Print and shaded views of the part. All mm, measured from the part's lowest x, y and z. A direction names the side the tool comes from. Round coordinates to 2 decimals unless told otherwise and drop trailing zeros. Order: outer loops, then holes, each group sorted by start corner. A loop starts at its lowest first (then second) coordinate and runs counter-clockwise, first axis right, second up. Notation, with made-up numbers: (-22, 42.25) - (35, 42.25) arc R21 cw to (35, 67.25) - close; hole circle Ø1 at (-36.5, 77). An arc over 180 degrees is marked (long way). Write item = value, one per line.
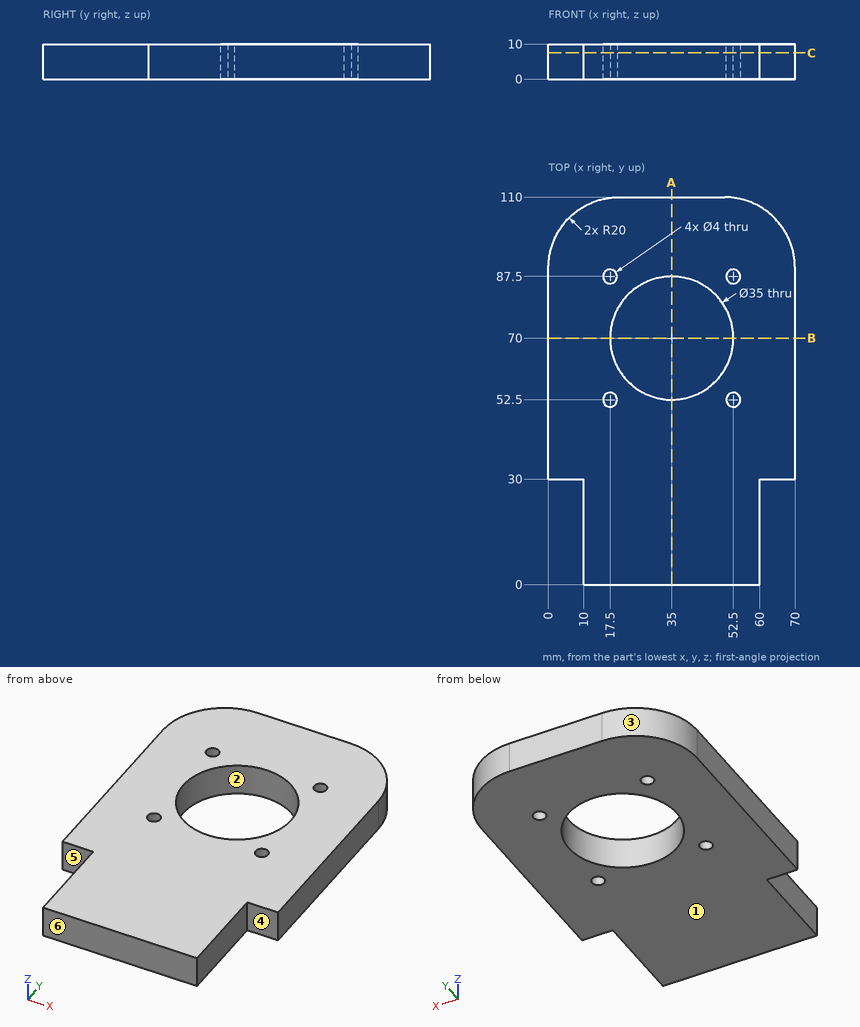
(1) Band-saw the part on B-B on y = 70. List the corners of the cut face in (x, z), plus the area to 3 significant figures.
Solved:
outline = (0, 0) - (17.5, 0) - (17.5, 10) - (0, 10) - close; (52.5, 0) - (70, 0) - (70, 10) - (52.5, 10) - close
area = 350 mm²
(2) Band-saw the part on C-C on z = 7.5. List the corners of the cut face in (x, y).
Solved:
outline = (0, 30) - (10, 30) - (10, 0) - (60, 0) - (60, 30) - (70, 30) - (70, 90) arc R20 ccw to (50, 110) - (20, 110) arc R20 ccw to (0, 90) - close; hole circle Ø4 at (17.5, 52.5); hole circle Ø4 at (17.5, 87.5); hole circle Ø35 at (35, 70); hole circle Ø4 at (52.5, 52.5); hole circle Ø4 at (52.5, 87.5)
(3) Pull direction X, two halves, no side cores. Call the marked faces 1, 2 and 3: released by +X, released by -X, zero draft, split by the parting line, or undercut.
Solved:
face_1 = zero draft
face_2 = undercut
face_3 = released by -X
(4) Band-saw the part on A-A on x = 35. List the corners of the cut face in (y, z).
Solved:
outline = (0, 0) - (52.5, 0) - (52.5, 10) - (0, 10) - close; (87.5, 0) - (110, 0) - (110, 10) - (87.5, 10) - close
(5) Drop flat-ended pins along their axis: pin 1 (5 mm diameter, centred on y = 16, z = 5, fed in from +X); pin 2 (2.5 mm diameter, centred on x = 52.5, y = 52.5, fed in from -Z); pin 3 (5 mm diameter, centred on y = 11, z = 7, fed in from -X). Give the stop position or say it passes through.
Solved:
pin_1 = 60
pin_2 = through
pin_3 = 10
(6) Tool access for the marked faces 4, 5 and 6: list every direction of +Z, -Z, +X, -X, +Y, -Y with a clear straight run to the whole face (end or side of a thin tool).
Solved:
face_4 = +Z, -Z, +X, -Y
face_5 = +Z, -Z, -X, -Y
face_6 = +Z, -Z, +X, -X, -Y
(7) Probe line 1 along X through (y, z) = (23.5, 4.75); line 2 along Y through (x, z) = (32.5, 7.75); line 3 along Y through (x, z) = (16.5, 4.5). List the from-to ranges inside material, lowest first.
Solved:
line_1 = 10 to 60
line_2 = 0 to 52.68, 87.32 to 110
line_3 = 0 to 50.77, 54.23 to 85.77, 89.23 to 109.69
